The listing builds one solid part. Answer for the finished solid, in the listing's coordinates (mm). A direction names the side the tool comes from. Give positions to 0.01 mm unless a question says otherwise; leave off trailing zeros. Write each loop counter-clockwise with the first axis right and the second up, starting at its lowest first coordinate (ties: lowest second). Pieces come first, ordered by that corner, then holes.
Autodesk Inventor part; units mm, degrees
ref_plane "YZ Plane" through (0, 0, 0) normal (1, 0, 0) x (0, 1, 0)
ref_plane "XZ Plane" through (0, 0, 0) normal (0, 1, 0) x (-1, 0, 0)
ref_plane "XY Plane" through (0, 0, 0) normal (0, 0, 1) x (1, 0, 0)
sketch "Náčrt1" plane through (0, 0, 0) normal (0, 1, 0) x (-1, 0, 0)
  line L0 (0, 0) -> (-106, 0)
  line L1 (-106, 0) -> (-106, -72)
  line L2 (-106, -72) -> (0, -72)
  line L3 (0, -72) -> (0, 0)
  dimension "d0" = 106
  dimension "d1" = 72
extrude "Vysunutí1" add sketch "Náčrt1" along normal blind 3
sketch "Náčrt2" plane through (0, 3, 0) normal (0, 1, 0) x (1, 0, 0)
  line L0 (0, 72) -> (0, 0)
  line L1 (106, 0) -> (106, 72)
  line L2 (0, 0) -> (106, 0)
  line L3 (106, 0) -> (106, 72)
  line L4 (106, 72) -> (0, 72)
  line L5 (0, 72) -> (0, 0)
  line L6 (2, 70) -> (104, 70)
  line L7 (104, 70) -> (104, 2)
  line L8 (104, 2) -> (2, 2)
  line L9 (2, 2) -> (2, 70)
  line L10 (2, 2) -> (8, 2)
  line L11 (8, 2) -> (8, 8)
  line L12 (8, 8) -> (2, 8)
  line L13 (2, 8) -> (2, 2)
  line L14 (2, 70) -> (8, 70)
  line L15 (8, 70) -> (8, 64)
  line L16 (8, 64) -> (2, 64)
  line L17 (2, 64) -> (2, 70)
  line L18 (53, -6.8672) -> (53, 83.3894) construction
  line L19 (104, 2) -> (104, 70)
  line L20 (104, 2) -> (98, 2)
  line L21 (98, 2) -> (98, 8)
  line L22 (98, 8) -> (104, 8)
  line L23 (104, 8) -> (104, 2)
  line L24 (104, 70) -> (98, 70)
  line L25 (98, 70) -> (98, 64)
  line L26 (98, 64) -> (104, 64)
  line L27 (104, 64) -> (104, 70)
  point P0 (2, 64)
  dimension "d4" = 2
  dimension "d5" = 6
  dimension "d6" = 6
  dimension "d7" = 6
  dimension "d8" = 6
extrude "Vysunutí2" add sketch "Náčrt2" along normal blind 10 contours L6 L15 L16 L9 | L6 L7 L26 L25 | L12 L11 L8 L9 | L7 L8 L21 L22
sketch "Náčrt3" plane through (2, 3, -2) normal (0, 0, 1) x (1, 0, 0)
  circle A0 centre (3, 6) radius 1.3
  line L0 (0, 10) -> (6, 10)
  line L1 (6, 0) -> (6, 10)
  line L2 (-2, 0) -> (104, 0)
  circle A1 centre (99, 6) radius 1.3
  line L3 (96, 10) -> (102, 10)
  line L4 (102, 0) -> (102, 10)
  point P0 (-2, -3)
  dimension "d11" = 2.6
  dimension "d12" = 4
  dimension "d13" = 3
  dimension "d14" = 6
  dimension "d15" = 2.6
  dimension "d16" = 4
  dimension "d17" = 3
  dimension "d18" = 6
extrude "Vysunutí3" cut sketch "Náčrt3" against normal blind 100
fillet "Zaoblení1" radius 2 20 edges at (106, 1.5, 0) (106, 1.5, -72) (0, 1.5, 0) (0, 1.5, -72) (2, 13, -67) (5, 13, -70) (8, 13, -67) (5, 13, -64) (8, 13, -5) (5, 13, -8) (2, 13, -5) (5, 13, -2) (98, 13, -5) (101, 13, -2) (104, 13, -5) (101, 13, -8) (104, 13, -67) (101, 13, -70) (98, 13, -67) (101, 13, -64)
equation "\"d6\" = d5"
equation "\"d7\" = d5"
equation "\"d8\" = d5"
properties part number "RPIholderTOP"
Item 1: A cutting plane is placed at A-A, the plane y = 6. Give the vertices of the cut face in (x, z).
Conclusion:
outline: (2, -70) - (8, -70) - (8, -64) - (2, -64) - close; (2, -8) - (8, -8) - (8, -2) - (2, -2) - close; (98, -70) - (104, -70) - (104, -64) - (98, -64) - close; (98, -8) - (104, -8) - (104, -2) - (98, -2) - close
Item 2: Each of these flat-tipped pins is pushed along its axis until it touches: P1, Ø8, axis at x = 25.5, z = -57, coming from the +Y side; P2, Ø1.5, axis at y = 4.5, z = -17, coming from the -X side; P3, Ø3, axis at x = 100.5, y = 5, coming from the -Z side; P4, Ø6.5, axis at x = 102, y = 9, coming from the +Z side. Where does it stop, or does it pass through?
Conclusion:
P1: stops at y = 3
P2: passes through
P3: stops at z = -70
P4: stops at z = -2
Item 3: Consider probe 1 along Y at (x, z) = (5, -4); probe 2 along Y at (x, z) = (67, -36.5). Determine where each line is inside the solid, lowest interval first.
Conclusion:
probe 1: y = 0 to 7.7, 10.3 to 13
probe 2: y = 0 to 3
Item 4: A cutting plane is placed at C-C, the plane z = -21. Give the vertices of the cut face in (x, y), plus the area to 3 significant figures.
Conclusion:
outline: (0, 0) - (106, 0) - (106, 3) - (0, 3) - close
area: 318 mm2
Item 5: A cutting plane is placed at B-B, the plane x = 83.5. Give the vertices of the cut face in (y, z), plus the area to 3 significant figures.
Conclusion:
outline: (0, -72) - (3, -72) - (3, 0) - (0, 0) - close
area: 216 mm2
Item 6: Which of the six approach directions +Z, -Z, +X, -X, +Y, -Y give full straight-line access (tool end or side, diameter ignored) to faces 1 (the face through (98.35, 12.13, -5.04)), 2 (the face through (2, 7, -5)), 3 (the face through (5, 12.2, -7.6)), 4 (the face through (54, 1, -72))?
Conclusion:
face 1: +Z, -Z, +Y
face 2: +Z, -Z, -X, +Y
face 3: +X, -X, +Y
face 4: -Z, +X, -X, +Y, -Y
Item 7: Determine the mould class of faces 5 (the face through (101.04, 12.13, -69.65)), 6 (the face through (2.35, 12.13, -67.04)), 7 (the face through (101.04, 12.13, -7.65)) for opening direction Z: pulls with the +Z half, pulls with the -Z half, needs draft (parallel to the pull), parting line crosses it, or undercut.
Conclusion:
face 5: pulls with the -Z half
face 6: needs draft
face 7: undercut
